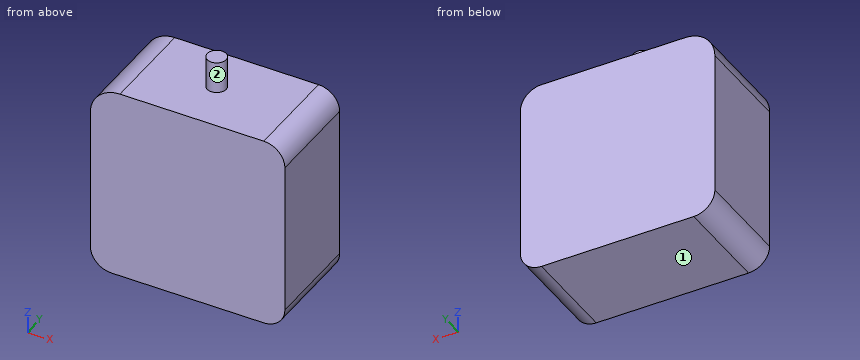
```python
from build123d import *

# Parameters (mm, degrees)
F0_W     = 46
F0_H     = 46
F1_DEPTH = 23
F2_R     = 7
F3_R     = 5
F4_R     = 2.25
F5_DEPTH = 7.5


with BuildPart() as f1:
    # F0 (on Front) → F1 (new body)
    with BuildSketch(Plane.XZ):
        Rectangle(F0_W, F0_H)
    extrude(amount=F1_DEPTH)

    # F2
    f2_edges = [f1.edges().sort_by_distance(p)[0] for p in [
        (-23, -11.5, 23),
    ]]
    fillet(f2_edges, radius=F2_R)

    # F3
    f3_edges = [f1.edges().sort_by_distance(p)[0] for p in [
        (23, -11.5, 23),
        (23, -11.5, -23),
        (-23, -11.5, -23),
    ]]
    fillet(f3_edges, radius=F3_R)

    # F4 (on face) → F5 (join)
    with BuildSketch(Plane.XY.offset(23)):
        with Locations((0, -10.782062)):
            Circle(F4_R)
    extrude(amount=F5_DEPTH)


solid = f1.part
```
Geometry check sheet. Reference: the model listing, model coordinates, mm. Face numbers are marked on the shaded views. A direction names the side the tool comes from. Round coordinates to 2 decimals unless told otherwise and drop trailing zeros. Order: outer loops, then holes, each group sorted by start corner. A loop starts at its lowest first (then second) coordinate and runs counter-clockwise, first axis right, second up. Notation, with made-up numbers: M 60,-20.75 L 79,-20.75 A27 cw 79,16.25 Z; hole C 24,31.25 d7. An arc over 180 degrees is marked long. Write item = value, one per line.
Q1. Section check A-A (y = -7.5). Enter the section's corners in (x, z).
Answer block:
outline = M -23,-18 A5 ccw -18,-23 L 18,-23 A5 ccw 23,-18 L 23,18 A5 ccw 18,23 L -16,23 A7 ccw -23,16 Z
Q2. Scan lines: line 1 (Z direction, x = 9, y = -4); line 2 (Z direction, x = -18, y = -19); line 3 (X direction, y = -3.5, z = 21). Record each from-to range of solid material in increasing order.
Answer block:
line_1 = -23 to 23
line_2 = -23 to 22.71
line_3 = -20.9 to 22
Q3. Depth check by flat-ended pin: pin 1 Ø3 at (y, z) = (-12.5, 25) entering from +X; pin 2 Ø1.5 at (y, z) = (-8, 23) entering from +X. Enter the tip coordinate at first touch or a pass-through.
Answer block:
pin_1 = 2.24
pin_2 = 20.63
Q4. Section check C-C (x = 8). Enter the section's corners in (y, z).
Answer block:
outline = M -23,-23 L 0,-23 L 0,23 L -23,23 Z
Q5. Section check D-D (y = -11.75). Enter the section's corners in (x, z), plus the area to 3 significant figures.
Answer block:
outline = M -23,-18 A5 ccw -18,-23 L 18,-23 A5 ccw 23,-18 L 23,18 A5 ccw 18,23 L 2.03,23 L 2.03,30.5 L -2.03,30.5 L -2.03,23 L -16,23 A7 ccw -23,16 Z
area = 2,120 mm^2
Q6. Section check B-B (x = 0). Enter the section's corners in (y, z), plus the area to 3 significant figures.
Answer block:
outline = M -23,-23 L 0,-23 L 0,23 L -8.53,23 L -8.53,30.5 L -13.03,30.5 L -13.03,23 L -23,23 Z
area = 1,090 mm^2
Q7. Set-up check for the marked faces 1 and 2: record each of +Z, -Z, +X, -X, +Y, -Y from which the full face is reachable in a straight line by a thin tool's end or side.
Answer block:
face_1 = -Z, +X, -X, +Y, -Y
face_2 = +Z
